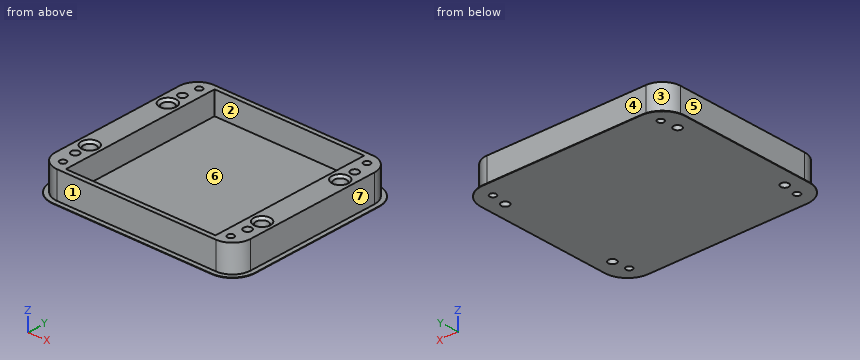
from build123d import *

# Parameters (mm, degrees)
F1_DEPTH = 2
F2_R     = 2.65
F2_W     = 65.6
F2_H     = 71.7
F3_DEPTH = 10
F4_R     = 1.4
F4_R_2   = 1.75
F5_DEPTH = 12
F6_SIZE  = 1
F8_DEPTH = 0.2


with BuildPart() as f1:
    # F0 (on Top) → F1 (new body)
    with BuildSketch(Plane.XY):
        with BuildLine():
            Line((34.8, 37.85), (-34.8, 37.85))
            ThreePointArc((-34.8, 37.85), (-40.456854, 35.506854), (-42.8, 29.85))
            Line((-42.8, 29.85), (-42.8, -29.85))
            ThreePointArc((-42.8, -29.85), (-40.456854, -35.506854), (-34.8, -37.85))
            Line((-34.8, -37.85), (34.8, -37.85))
            ThreePointArc((34.8, -37.85), (40.456854, -35.506854), (42.8, -29.85))
            Line((42.8, -29.85), (42.8, 29.85))
            ThreePointArc((42.8, 29.85), (40.456854, 35.506854), (34.8, 37.85))
        make_face()
    extrude(amount=F1_DEPTH)

    # F2 (on face) → F3 (join)
    with BuildSketch(Plane.XY.offset(2)):
        with BuildLine():
            ThreePointArc((-34.8, 37.85), (-40.456854, 35.506854), (-42.8, 29.85))
            Line((-42.8, 29.85), (-42.8, -29.85))
            ThreePointArc((-42.8, -29.85), (-40.456854, -35.506854), (-34.8, -37.85))
            Line((-34.8, -37.85), (34.8, -37.85))
            ThreePointArc((34.8, -37.85), (40.456854, -35.506854), (42.8, -29.85))
            Line((42.8, -29.85), (42.8, 29.85))
            ThreePointArc((42.8, 29.85), (40.456854, 35.506854), (34.8, 37.85))
            Line((34.8, 37.85), (-34.8, 37.85))
        make_face()
        with Locations((-37.8, -18.85)):
            Circle(F2_R, mode=Mode.SUBTRACT)
        with Locations((37.8, -18.85)):
            Circle(F2_R, mode=Mode.SUBTRACT)
        with Locations((-37.8, 18.85)):
            Circle(F2_R, mode=Mode.SUBTRACT)
        Rectangle(F2_W, F2_H, mode=Mode.SUBTRACT)
        with Locations((37.8, 18.85)):
            Circle(F2_R, mode=Mode.SUBTRACT)
    extrude(amount=F3_DEPTH)

    # F4 (on face) → F5 (cut, through all)
    with BuildSketch(Plane.XY.offset(12)):
        with Locations((-36.8, -32.85)):
            Circle(F4_R)
        with Locations((36.8, -32.85)):
            Circle(F4_R)
        with Locations((-36.8, 32.85)):
            Circle(F4_R)
        with Locations((36.8, 32.85)):
            Circle(F4_R)
        with Locations((-37.8, -25.85)):
            Circle(F4_R_2)
        with Locations((37.8, -25.85)):
            Circle(F4_R_2)
        with Locations((-37.8, 25.85)):
            Circle(F4_R_2)
        with Locations((37.8, 25.85)):
            Circle(F4_R_2)
    extrude(amount=-F5_DEPTH, mode=Mode.SUBTRACT)

    # F6
    f6_edges = [f1.edges().sort_by_distance(p)[0] for p in [
        (-40.45, 18.85, 12),
        (35.15, 18.85, 12),
        (35.15, -18.85, 12),
        (-40.45, -18.85, 12),
    ]]
    chamfer(f6_edges, length=F6_SIZE)

    # F7 (on face) → F8 (join)
    with BuildSketch(Plane(origin=(0, 0, 0), x_dir=(1, 0, 0), z_dir=(0, 0, -1))):
        with BuildLine():
            Line((34.8, 39.85), (-34.8, 39.85))
            ThreePointArc((-34.8, 39.85), (-41.871068, 36.921068), (-44.8, 29.85))
            Line((-44.8, 29.85), (-44.8, -29.85))
            ThreePointArc((-44.8, -29.85), (-41.871068, -36.921068), (-34.8, -39.85))
            Line((-34.8, -39.85), (34.8, -39.85))
            ThreePointArc((34.8, -39.85), (41.871068, -36.921068), (44.8, -29.85))
            Line((44.8, -29.85), (44.8, 29.85))
            ThreePointArc((44.8, 29.85), (41.871068, 36.921068), (34.8, 39.85))
        make_face()
        with BuildLine():
            Line((-42.8, -29.85), (-42.8, 29.85))
            ThreePointArc((-42.8, 29.85), (-40.456854, 35.506854), (-34.8, 37.85))
            Line((-34.8, 37.85), (34.8, 37.85))
            ThreePointArc((34.8, 37.85), (40.456854, 35.506854), (42.8, 29.85))
            Line((42.8, 29.85), (42.8, -29.85))
            ThreePointArc((42.8, -29.85), (40.456854, -35.506854), (34.8, -37.85))
            Line((34.8, -37.85), (-34.8, -37.85))
            ThreePointArc((-34.8, -37.85), (-40.456854, -35.506854), (-42.8, -29.85))
        make_face(mode=Mode.SUBTRACT)
    extrude(amount=-F8_DEPTH)


solid = f1.part
Here's how the part is built. I have some questions about the finished solid (model axes, mm). Face numbers are marked on the shaded views. A direction names the side the tool comes from. Give positions to 0.01 mm unless a question says otherwise; leave off trailing zeros. Order: outer loops, then holes, each group sorted by start corner. A loop starts at its lowest first (then second) coordinate and runs counter-clockwise, first axis right, second up. Notation, with made-up numbers: M 76,20 L 125,20 A12 ccw 125,28 Z; hole C 68.25,66 d9. An arc over 180 degrees is marked long. Answer as a JSON object with one key per item and string values. Group by question number.
1) We'd pull the mould along X, two halves only. Please class the marked faces 1, 2 and 3: pulls with the +X half, pulls with the -X half, needs draft (parallel to the pull), parting line crosses it, or undercut.
2) Please list where these lines run through material, in increasing order: L1, parallel to Y at x = -14.5, z = 6.5; L2, parallel to X at y = -25.5, z = 9; L3, parallel to Z at x = 3, y = 9. Write a range as [from, to].
3) Suppose I cut it at D-D, the plane y = 18.85. Write out the boundary of the cut face in (x, z), plus the area to 3 significant figures.
4) Suppose I cut it at B-B, the plane x = 20.5. Write out the boundary of the cut face in (y, z), plus the area to 3 significant figures.
5) I'm going to push flat-ended pins straight in: pin 1 Ø2.5 at (x, y) = (38, 19.5) entering from +Z; pin 2 Ø6 at (y, z) = (-11.5, 5.5) entering from -X; pin 3 Ø3.5 at (x, y) = (36.8, -32.85) entering from -Z; pin 4 Ø1 at (x, z) = (35.5, 7.5) entering from +Y. Where does each tip first touch, or does it pass through?
6) Suppose I cut it at A-A, the plane y = -25.85. Write out the boundary of the cut face in (x, z), plus the area to 3 significant figures.
7) On a 3-axis mill with a long thin cutter (end or side, diameter ignored), from which of +Z, -Z, +X, -X, +Y, -Y can I reach the whole of each face in a straight line? I mean the marked faces 4, 5, 6 and 7. Say none if no direction works.
8) Suppose I cut it at C-C, the plane z = 7.25. Count the separate pieces of the cut face and the enclosed holes in it, plus the area to 3 significant figures.
Results found:
{
 "1": {"face 1": "needs draft", "face 2": "undercut", "face 3": "pulls with the -X half"},
 "2": {"L1": "[-37.85, -35.85], [35.85, 37.85]", "L2": "[-42.8, -39.51], [-36.09, -32.8], [32.8, 36.09], [39.51, 42.8]", "L3": "[0, 2]"},
 "3": {"outline": "M -44.8,0 L 44.8,0 L 44.8,0.2 L 42.8,0.2 L 42.8,12 L 41.45,12 L 40.45,11 L 40.45,2 L 35.15,2 L 35.15,11 L 34.15,12 L 32.8,12 L 32.8,2 L -32.8,2 L -32.8,12 L -34.15,12 L -35.15,11 L -35.15,2 L -40.45,2 L -40.45,11 L -41.45,12 L -42.8,12 L -42.8,0.2 L -44.8,0.2 Z", "area": "264 mm²"},
 "4": {"outline": "M -39.85,0 L 39.85,0 L 39.85,0.2 L 37.85,0.2 L 37.85,12 L 35.85,12 L 35.85,2 L -35.85,2 L -35.85,12 L -37.85,12 L -37.85,0.2 L -39.85,0.2 Z", "area": "192 mm²"},
 "5": {"pin 1": "z = 2", "pin 2": "x = -42.8", "pin 3": "z = 0", "pin 4": "y = 37.85"},
 "6": {"outline": "M -44.8,0 L -39.55,0 L -39.55,12 L -42.8,12 L -42.8,0.2 L -44.8,0.2 Z; M -36.05,0 L 36.05,0 L 36.05,12 L 32.8,12 L 32.8,2 L -32.8,2 L -32.8,12 L -36.05,12 Z; M 39.55,0 L 44.8,0 L 44.8,0.2 L 42.8,0.2 L 42.8,12 L 39.55,12 Z", "area": "288 mm²"},
 "7": {"face 4": "+Z, +X, -X, +Y", "face 5": "+Z, -X, +Y, -Y", "face 6": "+Z", "face 7": "+Z, +X, +Y, -Y"},
 "8": {"separate pieces": "1", "enclosed holes": "13", "area": "1,570 mm²"}
}
